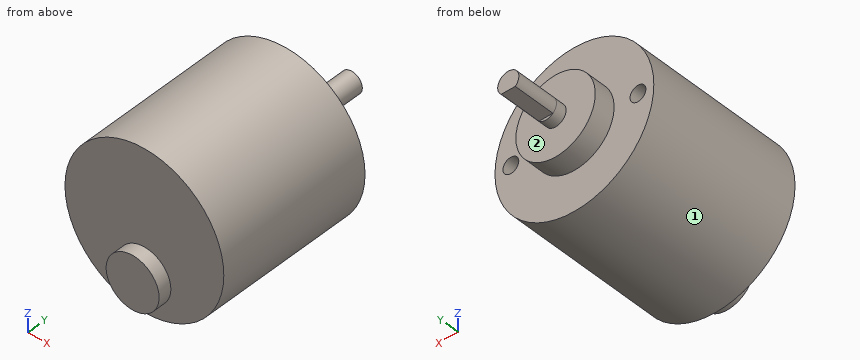
from build123d import *

# Parameters (mm, degrees)
SKETCH1_R           = 15
BOSS_EXTRUDE1_DEPTH = 30
SKETCH4_R           = 1.5
CUT_EXTRUDE1_DEPTH  = 4
SKETCH5_R           = 7.5
BOSS_EXTRUDE2_DEPTH = 4
SKETCH6_R           = 2
BOSS_EXTRUDE3_DEPTH = 2.05
BOSS_EXTRUDE4_DEPTH = 8
SKETCH9_R           = 5
BOSS_EXTRUDE5_DEPTH = 2.5


with BuildPart() as part:
    # Sketch1 → Boss-Extrude1 (new body)
    with BuildSketch(Plane(origin=(0, 0, 0), x_dir=(1, 0, 0), z_dir=(0, 1, 0))):
        Circle(SKETCH1_R)
    extrude(amount=BOSS_EXTRUDE1_DEPTH)

    # Sketch4 → Cut-Extrude1 (cut)
    with BuildSketch(Plane(origin=(0, 30, 0), x_dir=(1, 0, 0), z_dir=(0, 1, 0))):
        with Locations((12.005, 0)):
            Circle(SKETCH4_R)
        with Locations((-12.005, 0)):
            Circle(SKETCH4_R)
    extrude(amount=-CUT_EXTRUDE1_DEPTH, mode=Mode.SUBTRACT)

    # Sketch5 → Boss-Extrude2 (add)
    with BuildSketch(Plane(origin=(0, 30, 0), x_dir=(1, 0, 0), z_dir=(0, 1, 0))):
        Circle(SKETCH5_R)
    extrude(amount=BOSS_EXTRUDE2_DEPTH)

    # Sketch6 → Boss-Extrude3 (add)
    with BuildSketch(Plane(origin=(0, 34, 0), x_dir=(1, 0, 0), z_dir=(0, 1, 0))):
        Circle(SKETCH6_R)
    extrude(amount=BOSS_EXTRUDE3_DEPTH)

    # Sketch7 → Boss-Extrude4 (add)
    with BuildSketch(Plane(origin=(0, 36.05, 0), x_dir=(1, 0, 0), z_dir=(0, 1, 0))):
        with BuildLine():
            Line((-1.322875656, 1.5), (1.322875656, 1.5))
            ThreePointArc((1.322875656, 1.5), (0, -2), (-1.322875656, 1.5))
        make_face()
    extrude(amount=BOSS_EXTRUDE4_DEPTH)

    # Sketch9 → Boss-Extrude5 (add)
    with BuildSketch(Plane.XZ):
        with Locations((0, -8)):
            Circle(SKETCH9_R)
    extrude(amount=BOSS_EXTRUDE5_DEPTH)


solid = part.part
Input: part model. Units: mm. Frame: model coordinates. Face numbers are marked on the shaded views. A direction names the side the tool comes from. Give positions to 0.01 mm unless a question says otherwise; leave off trailing zeros. Write each loop counter-clockwise with the first axis right and the second up, starting at its lowest first coordinate (ties: lowest second). Pieces come first, ordered by that corner, then holes. Notation, with made-up numbers: M 83,6.25 L 132,6.25 A15 ccw 132,14.25 Z; hole C 19,22 d6. An arc over 180 degrees is marked long. Use one line per item in the form item = value.
1. Cut plane B-B on z = 0. Return loops of the section in (x, y) (3 decimals).
Outcome:
outline = M -15,0 L 15,0 L 15,30 L 13.505,30 L 13.505,26 L 10.505,26 L 10.505,30 L 7.5,30 L 7.5,34 L 2,34 L 2,44.05 L -2,44.05 L -2,34 L -7.5,34 L -7.5,30 L -10.505,30 L -10.505,26 L -13.505,26 L -13.505,30 L -15,30 Z
2. Cut plane D-D on z = -3.75. Return loops of the section in (x, y), and give its area (3 significant figures).
Outcome:
outline = M -14.52,0 L -2.63,0 L -2.63,-2.5 L 2.63,-2.5 L 2.63,0 L 14.52,0 L 14.52,30 L 6.5,30 L 6.5,34 L -6.5,34 L -6.5,30 L -14.52,30 Z
area = 937 mm²
3. Cut plane A-A on x = 0. Return loops of the section in (y, z), and give its area (3 significant figures).
Outcome:
outline = M -2.5,-13 L 0,-13 L 0,-15 L 30,-15 L 30,-7.5 L 34,-7.5 L 34,-2 L 36.05,-2 L 36.05,-1.5 L 44.05,-1.5 L 44.05,2 L 34,2 L 34,7.5 L 30,7.5 L 30,15 L 0,15 L 0,-3 L -2.5,-3 Z
area = 1,020 mm²
4. Reachability of the marked faces 1 and 2 from +Z, -Z, +X, -X, +Y, -Y: full face, straight path, thin tool, end or side. Return the list, or none.
Outcome:
face_1 = +Y, -Y
face_2 = +Y
5. Ray query, L1, parallel to X at y = 29.1, z = 0 (3 decimals); L2, parallel to Y at x = 7, z = 3.5; L3, parallel to Y at x = 0, z = 3.5. Return the intervals inside material, ascending.
Outcome:
L1 = -15 to -13.505, -10.505 to 10.505, 13.505 to 15
L2 = 0 to 30
L3 = 0 to 34
6. First-contact query: P1, Ø1.5, axis at x = -12, z = 0, coming from the +Y side; P2, Ø1, axis at y = 9.5, z = 11, coming from the -X side; P3, Ø3, axis at x = 7.5, y = 33, coming from the +Z side. Flat tips, straight axial feed; report the tip coordinate or a pass-through.
Outcome:
P1 = 26
P2 = -10.71
P3 = 4.5
7. Cut plane C-C on y = 17.5. Return loops of the section in (x, z), and give its area (3 significant figures).
Outcome:
outline = C 0,0 d30
area = 707 mm²
